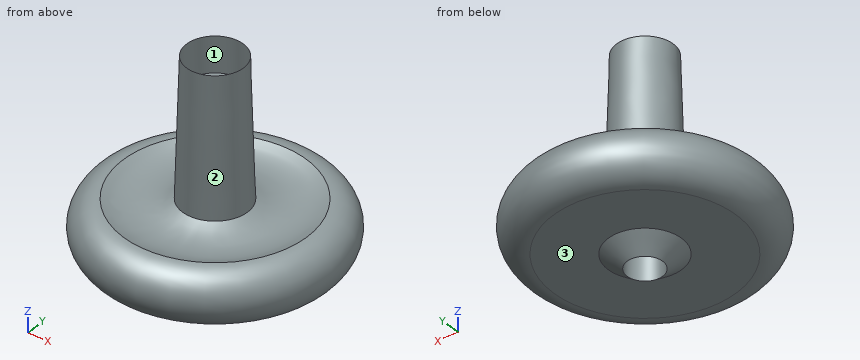
```python
from build123d import *

# Parameters (mm, degrees)
F2_R      = 4.7625
F1_FACE_R = 7.62
F3_DEPTH  = 9.525
F4_DEPTH  = 22.225


# Not quite as in the source:
# - a feature names something its author has since deleted; it is built from what else it names


with BuildPart() as f1:
    # F0 (on Front) → F1 (revolve)
    with BuildSketch(Plane.XZ):
        with BuildLine():
            Line((0, 58.42), (0, 0))
            Line((0, 0), (9.8843732849, 7.3464941233))
            Line((9.8843732849, 7.3464941233), (24.5773624629, 7.3464941233))
            ThreePointArc((24.5773624629, 7.3464941233), (31.75, 14.5191316605), (24.5773624629, 21.6917691976))
            ThreePointArc((24.5773624629, 21.6917691976), (16.6510342816, 19.7936922223), (8.7247061003, 21.6917691976))
            Line((8.7247061003, 21.6917691976), (7.62, 58.42))
            Line((7.62, 58.42), (0, 58.42))
        make_face()
    revolve(axis=Axis((0, 0, 29.21), (0, 0, -1)))

    # F2 (on Top) + F1_face (on face) → F3 (cut)
    with BuildSketch(Plane.XY):
        Circle(F2_R)
    with BuildSketch(Plane.XY.offset(58.42)):
        Circle(F1_FACE_R)
    extrude(amount=-F3_DEPTH, mode=Mode.SUBTRACT)

    # F2 (on Top) → F4 (cut)
    with BuildSketch(Plane.XY):
        Circle(F2_R)
    extrude(amount=F4_DEPTH, mode=Mode.SUBTRACT)


solid = f1.part
```
Input: part model. Units: mm. Frame: model coordinates. Face numbers are marked on the shaded views. Give positions to 0.01 mm unless a question says otherwise; leave off trailing zeros. Order: outer loops, then holes, each group sorted by start corner. A loop starts at its lowest first (then second) coordinate and runs counter-clockwise, first axis right, second up. Notation, with made-up numbers: M 72.25,6.25 L 123.25,6.25 A13 cw 123.25,20.25 Z; hole C 23.5,1.5 d1. An arc over 180 degrees is marked long. One line per question, with ' | ' between items.
1) Ray query, L1, parallel to Z at x = 11, y = -13.5; L2, parallel to Y at x = 0, z = 12; L3, parallel to Y at x = 0, z = 51.25. Return the intervals inside material, ascending.
Filled in:
L1: z = 7.35 to 19.81 | L2: y = -31.29 to -4.76, 4.76 to 31.29 | L3: y = -7.84 to -7.62, 7.62 to 7.84
2) Section B-B on z = 24. Output: boundary loops of the cut face in (x, y).
Filled in:
outline: C 0,0 d17.31
3) Draft query along X for the marked faces 1, 2 and 3. Return one class per face: pulls with the +X half, pulls with the -X half, needs draft (parallel to the pull), parting line crosses it, or undercut.
Filled in:
face 1: undercut | face 2: parting line crosses it | face 3: needs draft
4) Section A-A on z = 47. Output: boundary loops of the cut face in (x, y), and give its area (3 significant figures).
Filled in:
outline: C 0,0 d15.93 | area: 199 mm2
5) Contact query for flat-ended pins moving along their axis: P1, Ø7.5, axis at x = 0, y = 0, coming from the -Z side (3 decimals); P2, Ø4, axis at y = 9.5, z = 25.5, coming from the -X side; P3, Ø17, axis at x = -1.5, y = 2.5, coming from the +Z side; P4, Ø8, axis at x = 1, y = 11.5, coming from the -Z side. Output: stop coordinate, or through.
Filled in:
P1: stops at z = 22.225 | P2: stops at x = -4.23 | P3: stops at z = 58.42 | P4: stops at z = 5.61
